Read the model definition and answer for the solid it produces. Units are mm, in the model's axes. Coordinates: 2 decimals unless noted, no trailing zeros. Write each loop counter-clockwise with the first axis right and the second up, starting at its lowest first coordinate (ties: lowest second). Pieces come first, ordered by that corner, then holes.
(1) Find the intervals of material crossed by probe 1 along Y at (x, z) = (-19.5, 0.25); probe 2 along X at (y, z) = (19.5, 2.75), in increasing order.
(2) Section A-A on y = 20.75 is taken. Write down the section's boundary in (x, z).
(3) Given pin 1 (4 mm diameter, centred on x = 5.5, z = 2, fed in from -Y); pin 2 (2.5 mm diameter, centred on x = -19.5, y = 2.25, fed in from +Z), each flat-ended and moving along its own axis, determine where each tip first touches the part or whether it passes through.
(4) Section B-B on x = -19.5 is taken. Write down the section's boundary in (y, z), then the cut area to 3 significant figures.
from build123d import *

# Parameters (mm, degrees)
SKETCH2_W           = 45
SKETCH2_H           = 10
BOSS_EXTRUDE1_DEPTH = 40
SKETCH3_R           = 1.45
CUT_EXTRUDE1_DEPTH  = 40
SKETCH4_W           = 45
SKETCH4_H           = 10
BOSS_EXTRUDE2_DEPTH = 10


with BuildPart() as part:
    # Sketch2 → Boss-Extrude1 (new body)
    with BuildSketch(Plane(origin=(0, 0, 0), x_dir=(1, 0, 0), z_dir=(0, 1, 0))):
        Rectangle(SKETCH2_W, SKETCH2_H)
    extrude(amount=BOSS_EXTRUDE1_DEPTH)

    # Sketch3 → Cut-Extrude1 (cut)
    with BuildSketch(Plane(origin=(0, 0, -5), x_dir=(-1, 0, 0), z_dir=(0, 0, -1))):
        with Locations((19.5, 2.25)):
            Circle(SKETCH3_R)
        with Locations((-19.5, 2.25)):
            Circle(SKETCH3_R)
        with Locations((-19.5, 20.75)):
            Circle(SKETCH3_R)
        with Locations((19.5, 20.75)):
            Circle(SKETCH3_R)
    extrude(amount=-CUT_EXTRUDE1_DEPTH, mode=Mode.SUBTRACT)

    # Sketch4 → Boss-Extrude2 (add)
    with BuildSketch(Plane(origin=(0, 40, 0), x_dir=(1, 0, 0), z_dir=(0, 1, 0))):
        Rectangle(SKETCH4_W, SKETCH4_H)
    extrude(amount=BOSS_EXTRUDE2_DEPTH)


solid = part.part
Response:
1. probe 1: y = 0 to 0.8, 3.7 to 19.3, 22.2 to 50
1. probe 2: x = -22.5 to -20.23, -18.77 to 18.77, 20.23 to 22.5
2. outline: (-22.5, -5) - (-20.95, -5) - (-20.95, 5) - (-22.5, 5) - close; (-18.05, -5) - (18.05, -5) - (18.05, 5) - (-18.05, 5) - close; (20.95, -5) - (22.5, -5) - (22.5, 5) - (20.95, 5) - close
3. pin 1: stops at y = 0
3. pin 2: passes through
4. outline: (0, -5) - (0.8, -5) - (0.8, 5) - (0, 5) - close; (3.7, -5) - (19.3, -5) - (19.3, 5) - (3.7, 5) - close; (22.2, -5) - (50, -5) - (50, 5) - (22.2, 5) - close
4. area: 442 mm2
